Input: part model. Units: mm. Frame: model coordinates. Face numbers are marked on the shaded views. A direction names the side the tool comes from. Round coordinates to 2 decimals unless told otherwise and drop trailing zeros. Order: outer loops, then holes, each group sorted by start corner. A loop starts at its lowest first (then second) coordinate and runs counter-clockwise, first axis right, second up. Notation, with made-up numbers: (37, -30) -> (46, -30) arc R23 cw to (46, -17) -> close; hole circle Ø6 at (84, 19). An arc over 180 degrees is marked (long way). Use a Markdown table: item, result.
Autodesk Inventor part; units mm, degrees
ref_plane "YZ Plane" through (0, 0, 0) normal (1, 0, 0) x (0, 1, 0)
ref_plane "XZ Plane" through (0, 0, 0) normal (0, 1, 0) x (-1, 0, 0)
ref_plane "XY Plane" through (0, 0, 0) normal (0, 0, 1) x (1, 0, 0)
sketch "Sketch1" plane through (0, 0, 0) normal (0, 0, 1) x (1, 0, 0)
  line L0 (0, 3.6903) -> (0, -33.2554)
  line L1 (0, 0) -> (5.5, 0)
  line L2 (5.5, 0) -> (5.5, -10)
  line L3 (5.5, -10) -> (8.5, -10)
  line L4 (8.5, -10) -> (8.5, 0)
  line L5 (8.5, 0) -> (19.5, 0)
  line L6 (19.5, 0) -> (19.5, -30)
  line L7 (19.5, -30) -> (8.5, -30)
  line L8 (8.5, -30) -> (8.5, -20)
  line L9 (8.5, -20) -> (5.5, -20)
  line L10 (5.5, -20) -> (5.5, -30)
  line L11 (0, -30) -> (5.5, -30)
  line L12 (0, 0) -> (-5.5, 0)
  line L13 (-5.5, 0) -> (-5.5, -10)
  line L14 (-5.5, -10) -> (-8.5, -10)
  line L15 (-8.5, -10) -> (-8.5, 0)
  line L16 (-8.5, 0) -> (-19.5, 0)
  line L17 (-19.5, 0) -> (-19.5, -30)
  line L18 (-19.5, -30) -> (-8.5, -30)
  line L19 (-8.5, -30) -> (-8.5, -20)
  line L20 (-8.5, -20) -> (-5.5, -20)
  line L21 (-5.5, -20) -> (-5.5, -30)
  line L22 (0, -30) -> (-5.5, -30)
  dimension "d0" = 5.5
  dimension "d1" = 10
  dimension "d2" = 3
  dimension "d3" = 11
  dimension "d4" = 30
  dimension "d5" = 11
  dimension "d6" = 10
  dimension "d7" = 5.5
  dimension "d8" = 3
extrude "Extrusion1" add sketch "Sketch1" along normal blind 23
equation "\"d5\" = d3"
equation "\"d6\" = d1"
equation "\"d7\" = d0"
equation "\"d8\" = d2"
properties part number "CommonGNDVDD" material "ABS Plastic"
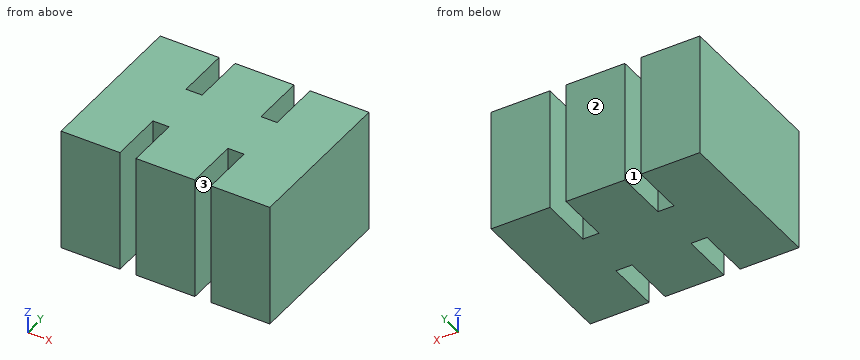
1) Ray query, probe 1 along X at (y, z) = (-21.25, 15.5); probe 2 along Y at (x, z) = (7.5, 15.75). Return the intervals inside material, ascending.
Answer key:
| item | result |
|---|---|
| probe 1 | x = -19.5 to -8.5, -5.5 to 5.5, 8.5 to 19.5 |
| probe 2 | y = -20 to -10 |
2) Cut plane A-A on y = -22. Return loops of the section in (x, z).
Answer key:
| item | result |
|---|---|
| outline | (-19.5, 0) -> (-8.5, 0) -> (-8.5, 23) -> (-19.5, 23) -> close; (-5.5, 0) -> (5.5, 0) -> (5.5, 23) -> (-5.5, 23) -> close; (8.5, 0) -> (19.5, 0) -> (19.5, 23) -> (8.5, 23) -> close |
3) Cut plane B-B on z = 20.75. Return loops of the section in (x, y).
Answer key:
| item | result |
|---|---|
| outline | (-19.5, -30) -> (-8.5, -30) -> (-8.5, -20) -> (-5.5, -20) -> (-5.5, -30) -> (5.5, -30) -> (5.5, -20) -> (8.5, -20) -> (8.5, -30) -> (19.5, -30) -> (19.5, 0) -> (8.5, 0) -> (8.5, -10) -> (5.5, -10) -> (5.5, 0) -> (-5.5, 0) -> (-5.5, -10) -> (-8.5, -10) -> (-8.5, 0) -> (-19.5, 0) -> close |
4) Cut plane C-C on x = -7. Return loops of the section in (y, z), and give its area (3 significant figures).
Answer key:
| item | result |
|---|---|
| outline | (-20, 0) -> (-10, 0) -> (-10, 23) -> (-20, 23) -> close |
| area | 230 mm^2 |
5) Set-up query: the marked faces 1, 2 and 3. Return all of +Z, -Z, +X, -X, +Y, -Y with unobstructed straight access to the full face (end or side cutting, diameter ignored); none if empty.
Answer key:
| item | result |
|---|---|
| face 1 | +Z, -Z, +Y |
| face 2 | +Z, -Z, +X, -X, +Y |
| face 3 | +Z, -Z, -Y |
6) Contact query for flat-ended pins moving along their axis: P1, Ø2.5, axis at x = 6.5, z = 17, coming from the +Y side; P2, Ø1.5, axis at x = -7, z = 17, coming from the +Y side; P3, Ø0.9, axis at x = 7.5, z = 6.5, coming from the -Y side. Output: stop coordinate, or through.
Answer key:
| item | result |
|---|---|
| P1 | stops at y = 0 |
| P2 | stops at y = -10 |
| P3 | stops at y = -20 |
